Source: three-view drawing plus pictorial views. Frame: mm from the lowest corner of the part. A direction names the side the tool comes from. Give positions to 0.01 mm unless a question says otherwise; leave off trailing zeros. Loops run counter-clockwise (first coordinate to the right, second up) from the corner with the lowest first, then second, coordinate; pieces in that order, holes last. Notation, with made-up numbers: (82, 33) - (93, 33) arc R29 ccw to (93, 63) - close; hole circle Ø6 at (14, 23). An arc over 180 degrees is marked (long way). One line per item, written item: value.
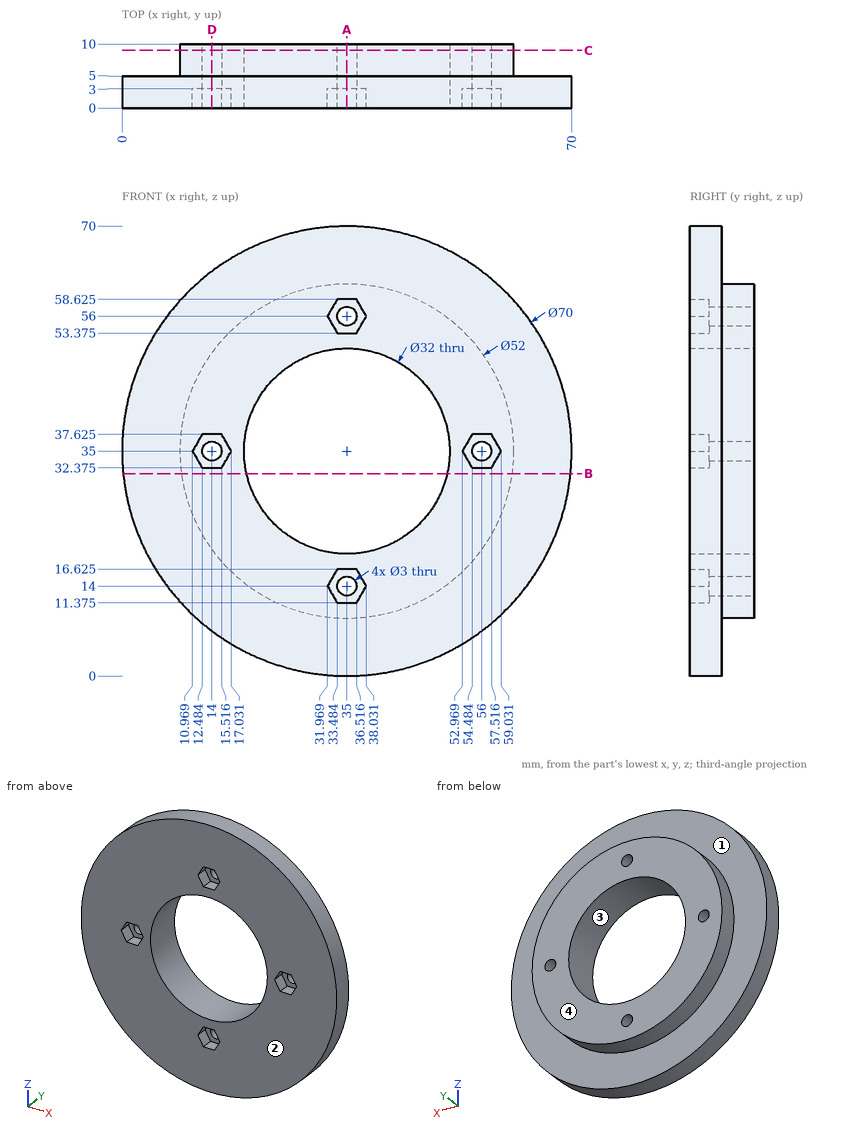
Item 1: Pin query (flat end, axial travel): P1, Ø2, axis at x = 9, y = 2.5, coming from the +Z side (1 decimal); P2, Ø2.5, axis at x = 35, y = 2, coming from the -Z side; P3, Ø5, axis at y = 8, z = 42, coming from the +X side. Return the tip coordinate at first contact, or that it passes through.
Verdict:
P1: stops at z = 59.5
P2: stops at z = 0
P3: stops at x = 60.61
Item 2: Access query for the marked faces 1 and 2. Directions: +Z, -Z, +X, -X, +Y, -Y. A direction counts if a zero-diameter tool reaches every point of the face in a straight line with its end or side. Return the directions, or none.
Verdict:
face 1: +Y
face 2: +Z, -Z, +X, -X, -Y
Item 3: Section C-C, the plane y = 9. Output: boundary loops of the cut face in (x, z), and give its area (3 significant figures).
Verdict:
outline: circle Ø52 at (35, 35); hole circle Ø3 at (14, 35); hole circle Ø32 at (35, 35); hole circle Ø3 at (35, 14); hole circle Ø3 at (35, 56); hole circle Ø3 at (56, 35)
area: 1,290 mm^2
Item 4: Section B-B, the plane z = 31.5. Output: boundary loops of the cut face in (x, y) (1 decimal), and give its area (3 significant figures).
Verdict:
outline: (0.2, 0) - (19.4, 0) - (19.4, 10) - (9.2, 10) - (9.2, 5) - (0.2, 5) - close; (50.6, 0) - (69.8, 0) - (69.8, 5) - (60.8, 5) - (60.8, 10) - (50.6, 10) - close
area: 294 mm^2
Item 5: Section A-A, the plane x = 35. Output: boundary loops of the cut face in (y, z) (1 decimal).
Verdict:
outline: (0, 0) - (5, 0) - (5, 9) - (10, 9) - (10, 12.5) - (3, 12.5) - (3, 11.4) - (0, 11.4) - close; (0, 16.6) - (3, 16.6) - (3, 15.5) - (10, 15.5) - (10, 19) - (0, 19) - close; (0, 51) - (10, 51) - (10, 54.5) - (3, 54.5) - (3, 53.4) - (0, 53.4) - close; (0, 58.6) - (3, 58.6) - (3, 57.5) - (10, 57.5) - (10, 61) - (5, 61) - (5, 70) - (0, 70) - close
Item 6: Draft query along Z for the marked faces 3 and 4. Return one class per face: pulls with the +Z half, pulls with the -Z half, needs draft (parallel to the pull), parting line crosses it, or undercut.
Verdict:
face 3: undercut
face 4: needs draft
Item 7: Material intervals for L1, parallel to X at y = 8.25, z = 35; L2, parallel to Z at x = 36.5, y = 1.75 (1 decimal), sorted ascending.
Verdict:
L1: x = 9 to 12.5, 15.5 to 19, 51 to 54.5, 57.5 to 61
L2: z = 0 to 11.4, 16.6 to 19.1, 50.9 to 53.4, 58.6 to 70
Item 8: Section D-D, the plane x = 14. Output: boundary loops of the cut face in (y, z) (1 decimal).
Verdict:
outline: (0, 7) - (5, 7) - (5, 19.7) - (10, 19.7) - (10, 33.5) - (3, 33.5) - (3, 32.4) - (0, 32.4) - close; (0, 37.6) - (3, 37.6) - (3, 36.5) - (10, 36.5) - (10, 50.3) - (5, 50.3) - (5, 63) - (0, 63) - close
